Geometry: final body of the model. Coordinates: model frame, mm. Face numbers are marked on the shaded views. A direction names the side the tool comes from. Give positions to 0.01 mm unless a question says otherwise; leave off trailing zeros. Write each loop counter-clockwise with the first axis right and the second up, starting at its lowest first coordinate (ties: lowest second). Pieces come first, ordered by that corner, then holes.
Q1. Section A-A (z = 16). Return the cut outline in (x, y), plus the area to 3 significant figures.
Q2. Pin query (flat end, axial travel): pin 1 Ø8 at (x, y) = (38, -5) entering from +Z; pin 2 Ø6 at (x, y) = (7, -3) entering from +Z; pin 3 Ø2 at (y, z) = (2.5, 2) entering from -X; pin 4 Ø4 at (y, z) = (3, 9.5) entering from +X. Return the tip coordinate at first contact, or that it passes through.
Q3. Section C-C (y = 0). Return the cut outline in (x, z).
Q4. Section D-D (y = -5). Return the cut outline in (x, z).
Q5. Line query: line 1 (Y direction, x = 9, z = 1); line 2 (X direction, y = 1.75, z = 2.5); line 3 (X direction, y = -3.25, z = 8). Output: solid intervals per line, ascending.
Q6. Reachability of the marked faces 1, 2 and 3 from +Z, -Z, +X, -X, +Y, -Y: full face, straight path, thin tool, end or side. Return the list, or none.
Q7. Mould query, pull axis X, two halves, no side actions, for the marked faces 4, 5, 6 and 7. Classes: +X half, -X half, draft (parallel to the pull), parting line (faces both ways), or undercut.
Q8. Section B-B (x = -18). Return the cut outline in (y, z), plus the area to 3 significant figures.
from build123d import *

# Parameters (mm, degrees)
ESQUISSE1_W             = 5
ESQUISSE1_H             = 24
ESQUISSE1_W_2           = 96
ESQUISSE1_W_3           = 70
ESQUISSE1_H_2           = 16
BOSS_EXTRU_1_DEPTH      = 4
ESQUISSE2_W             = 5
ESQUISSE2_H             = 24
BOSS_EXTRU_2_DEPTH      = 8.75
BOSS_EXTRU_3_DEPTH      = 5
ESQUISSE4_R             = 1.75
ENL_V_MAT_EXTRU_2_DEPTH = 18.75


with BuildPart() as part:
    # Esquisse1 → Boss.-Extru.1 (new body)
    with BuildSketch(Plane.XY):
        with Locations((-50.5, 0)):
            Rectangle(ESQUISSE1_W, ESQUISSE1_H)
        Rectangle(ESQUISSE1_W_2, ESQUISSE1_H)
        Rectangle(ESQUISSE1_W_3, ESQUISSE1_H_2, mode=Mode.SUBTRACT)
        with Locations((50.5, 0)):
            Rectangle(ESQUISSE1_W, ESQUISSE1_H)
    extrude(amount=BOSS_EXTRU_1_DEPTH)

    # Esquisse2 → Boss.-Extru.2 (add)
    with BuildSketch(Plane.XY.offset(4)):
        with Locations((-50.5, 0)):
            Rectangle(ESQUISSE2_W, ESQUISSE2_H)
        with Locations((50.5, 0)):
            Rectangle(ESQUISSE2_W, ESQUISSE2_H)
    extrude(amount=BOSS_EXTRU_2_DEPTH)

    # Esquisse3 → Boss.-Extru.3 (add)
    with BuildSketch(Plane.XY.offset(12.75)):
        with BuildLine():
            Line((-48, 12), (-53, 12))
            ThreePointArc((-53, 12), (-63, 0), (-53, -12))
            Line((-53, -12), (-48, -12))
            Line((-48, -12), (-48, 12))
        make_face()
        with BuildLine():
            Line((48, -12), (53, -12))
            ThreePointArc((53, -12), (63, 0), (53, 12))
            Line((53, 12), (48, 12))
            Line((48, 12), (48, -12))
        make_face()
    extrude(amount=BOSS_EXTRU_3_DEPTH)

    # Esquisse4 → Enlèv. mat.-Extru.2 (cut, through all)
    with BuildSketch(Plane.XY.offset(17.75)):
        with Locations((-58, 0)):
            Circle(ESQUISSE4_R)
        with Locations((58, 0)):
            Circle(ESQUISSE4_R)
    extrude(amount=-ENL_V_MAT_EXTRU_2_DEPTH, mode=Mode.SUBTRACT)


solid = part.part
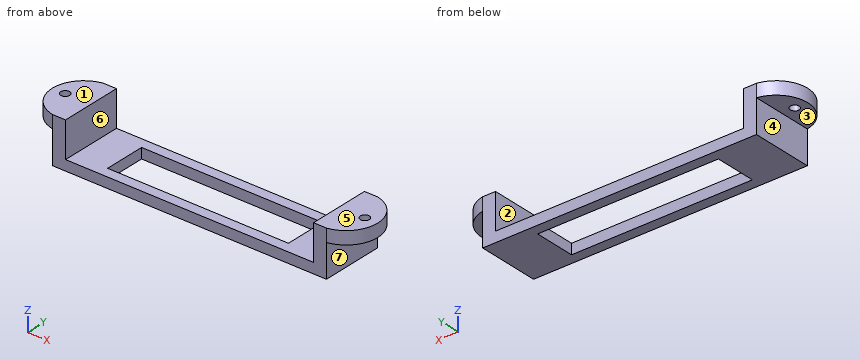
Computed:
1. outline: (-53, -12) - (-48, -12) - (-48, 12) - (-53, 12) arc R12.2 ccw to start; (48, -12) - (53, -12) arc R12.2 ccw to (53, 12) - (48, 12) - close; hole circle Ø3.5 at (-58, 0); hole circle Ø3.5 at (58, 0)
1. area: 582 mm2
2. pin 1: stops at z = 4
2. pin 2: passes through
2. pin 3: stops at x = -53
2. pin 4: stops at x = 53
3. outline: (-63, 12.75) - (-59.75, 12.75) - (-59.75, 17.75) - (-63, 17.75) - close; (-56.25, 12.75) - (-53, 12.75) - (-53, 0) - (-35, 0) - (-35, 4) - (-48, 4) - (-48, 17.75) - (-56.25, 17.75) - close; (35, 0) - (53, 0) - (53, 12.75) - (56.25, 12.75) - (56.25, 17.75) - (48, 17.75) - (48, 4) - (35, 4) - close; (59.75, 12.75) - (63, 12.75) - (63, 17.75) - (59.75, 17.75) - close
4. outline: (-61.93, 12.75) - (-53, 12.75) - (-53, 0) - (-35, 0) - (-35, 4) - (-48, 4) - (-48, 17.75) - (-61.93, 17.75) - close; (35, 0) - (53, 0) - (53, 12.75) - (61.93, 12.75) - (61.93, 17.75) - (48, 17.75) - (48, 4) - (35, 4) - close
5. line 1: y = -12 to -8, 8 to 12
5. line 2: x = -53 to -35, 35 to 53
5. line 3: x = -53 to -48, 48 to 53
6. face 1: +Z, +X, -X, +Y, -Y
6. face 2: +Z, +Y, -Y
6. face 3: -Z, -X, +Y, -Y
7. face 4: -X half
7. face 5: draft
7. face 6: undercut
7. face 7: +X half
8. outline: (-12, 0) - (-8, 0) - (-8, 4) - (-12, 4) - close; (8, 0) - (12, 0) - (12, 4) - (8, 4) - close
8. area: 32.0 mm2
